Design review of the part shown in the three views and the two pictorial views. Dimensions are in mm from the part's minimum x, y and z. A direction names the side the tool comes from. Round coordinates to 2 decimals unless told otherwise and drop trailing zeros. Write each loop counter-clockwise with the first axis right and the second up, starting at its lowest first coordinate (ties: lowest second). Pieces come first, ordered by that corner, then holes. Notation, with made-up numbers: (-35, 30.25) - (-2, 30.25) arc R28 ccw to (-2, 53.25) - close; hole circle Ø7 at (-23, 24.25). An arc over 180 degrees is marked (long way). One line per item, written item: value. Start each with the question number.
Q1. Tool access review of the marked faces 1 and 2: name each direction out of +Z, -Z, +X, -X, +Y, -Y from which nothing blocks a thin tool from reaching the whole face with its end or side.
Q2. Add section D-D on z = 15.5. Write out the cut boundary in (x, y).
Q3. Mouldability with a two-part tool opening along Z and no side actions: class the marked faces 3, 4 and 5 as +Z half, -Z half, draft (parallel to the pull), parting line (faces both ways), or undercut.
Q4. Clearance check with flat-ended pins moving along their axes: pin 1 Ø5 at (x, y) = (3.5, 7) entering from -Z; pin 2 Ø2 at (x, z) = (4.5, 15) entering from -Y; pin 3 Ø5 at (x, z) = (3.5, 11) entering from -Y. State where each tip first meets the part, or that it passes through.
Q5. For probe 1 along Z at (x, y) = (3, 11); probe 2 along Y at (x, z) = (10.25, 11); probe 3 along X at (y, z) = (18.5, 13), list the stretches that pass through material, from the lowest coordinate up.
Q6. Add section A-A on z = 11. Write out the cut boundary in (x, y).
Q7. Add section C-C on x = 5.75. Write out the cut boundary in (y, z), and give its area (3 significant figures).
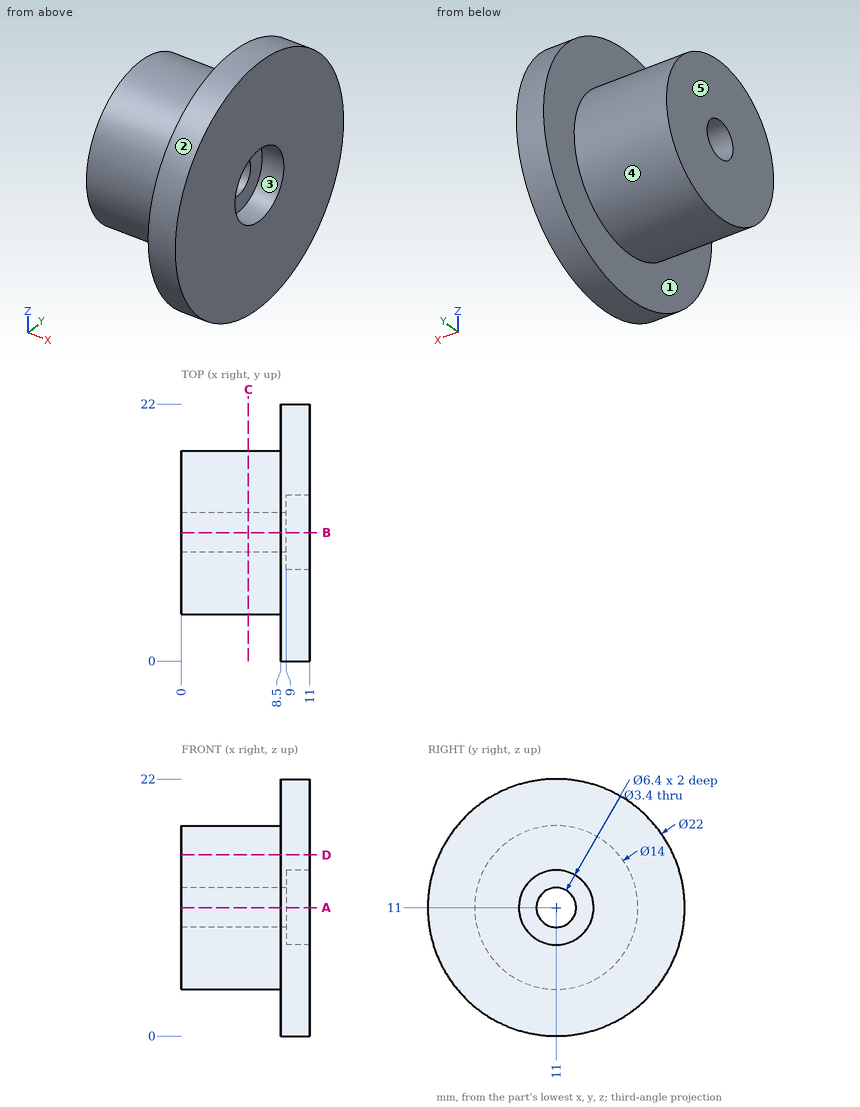
Result set:
1. face 1: -X
1. face 2: +X, -X
2. outline: (0, 5.64) - (8.5, 5.64) - (8.5, 0.96) - (11, 0.96) - (11, 21.04) - (8.5, 21.04) - (8.5, 16.36) - (0, 16.36) - close
3. face 3: undercut
3. face 4: parting line
3. face 5: draft
4. pin 1: stops at z = 4.16
4. pin 2: stops at y = 4.68
4. pin 3: stops at y = 4
5. probe 1: z = 4 to 9.3, 12.7 to 18
5. probe 2: y = 0 to 7.8, 14.2 to 22
5. probe 3: x = 8.5 to 11
6. outline: (0, 4) - (8.5, 4) - (8.5, 0) - (11, 0) - (11, 7.8) - (9, 7.8) - (9, 9.3) - (0, 9.3) - close; (0, 12.7) - (9, 12.7) - (9, 14.2) - (11, 14.2) - (11, 22) - (8.5, 22) - (8.5, 18) - (0, 18) - close
7. outline: circle Ø14 at (11, 11); hole circle Ø3.4 at (11, 11)
7. area: 145 mm^2
